Geometry: final body of the model. Coordinates: model frame, mm. Face numbers are marked on the shaded views. A direction names the side the tool comes from. Give positions to 0.01 mm unless a question says otherwise; leave off trailing zeros. Loops run counter-clockwise (first coordinate to the right, second up) from the corner with the lowest first, then second, coordinate; pieces in that order, holes last. Notation, with made-up numbers: (44, 48) - (67, 48) arc R25 ccw to (67, 81) - close; hole circle Ø4 at (75.25, 71). An arc over 180 degrees is marked (long way). Answer in a Markdown table with one row per item.
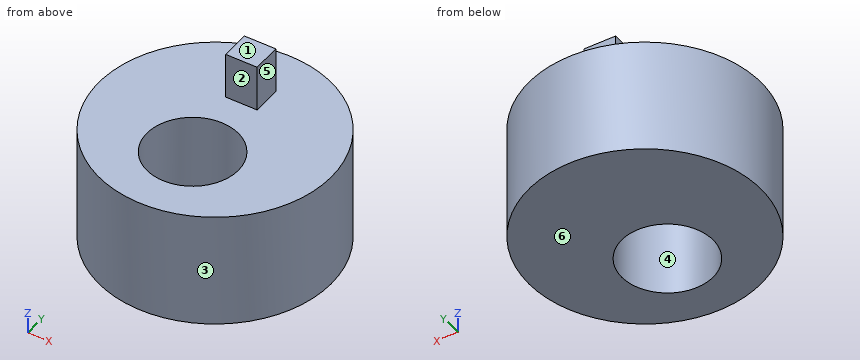
from build123d import *

# Parameters (mm, degrees)
SKETCH1_R           = 6.35
SKETCH1_R_2         = 2.499995
BOSS_EXTRUDE1_DEPTH = 6.35
SKETCH2_W           = 1.71989263
SKETCH2_H           = 1.584620177
BOSS_EXTRUDE2_DEPTH = 2.54


with BuildPart() as part:
    # Sketch1 → Boss-Extrude1 (new body)
    with BuildSketch(Plane.XY):
        Circle(SKETCH1_R)
        with Locations((0, -1.905)):
            Circle(SKETCH1_R_2, mode=Mode.SUBTRACT)
    extrude(amount=BOSS_EXTRUDE1_DEPTH)

    # Sketch2 → Boss-Extrude2 (add)
    with BuildSketch(Plane.XY.offset(6.35)):
        with Locations((-0.009662318, 3.043630217)):
            Rectangle(SKETCH2_W, SKETCH2_H)
    extrude(amount=BOSS_EXTRUDE2_DEPTH)


solid = part.part
Q1. Cut plane C-C (z = 6.75). Output: boundary loops of the cut face in (x, y), and give its area (3 significant figures).
Check values:
| item | result |
|---|---|
| outline | (-0.87, 2.25) - (0.85, 2.25) - (0.85, 3.84) - (-0.87, 3.84) - close |
| area | 2.73 mm² |
Q2. Cut plane D-D (y = 3.25). Output: boundary loops of the cut face in (x, z).
Check values:
| item | result |
|---|---|
| outline | (-5.46, 0) - (5.46, 0) - (5.46, 6.35) - (0.85, 6.35) - (0.85, 8.89) - (-0.87, 8.89) - (-0.87, 6.35) - (-5.46, 6.35) - close |
Q3. Draft query along X for the marked faces 3, 4, 5 and 6. Return one class per face: pulls with the +X half, pulls with the -X half, needs draft (parallel to the pull), parting line crosses it, or undercut.
Check values:
| item | result |
|---|---|
| face 3 | parting line crosses it |
| face 4 | undercut |
| face 5 | pulls with the +X half |
| face 6 | needs draft |
Q4. First-contact query: pin 1 (3 mm diameter, centred on x = -4.5, z = 5.5, fed in from -Y); pin 2 (0.9 mm diameter, centred on x = -0.5, z = 7.5, fed in from -Y); pin 3 (1.7 mm diameter, centred on y = 3, z = 7.5, fed in from -X). Flat tips, straight axial feed; report the tip coordinate or a pass-through.
Check values:
| item | result |
|---|---|
| pin 1 | y = -5.6 |
| pin 2 | y = 2.25 |
| pin 3 | x = -0.87 |
Q5. Cut plane A-A (x = 0). Output: boundary loops of the cut face in (y, z) (3 decimals), and give its area (3 significant figures).
Check values:
| item | result |
|---|---|
| outline | (-6.35, 0) - (-4.405, 0) - (-4.405, 6.35) - (-6.35, 6.35) - close; (0.595, 0) - (6.35, 0) - (6.35, 6.35) - (3.836, 6.35) - (3.836, 8.89) - (2.251, 8.89) - (2.251, 6.35) - (0.595, 6.35) - close |
| area | 52.9 mm² |
Q6. Cut plane B-B (y = -0.25). Output: boundary loops of the cut face in (x, z).
Check values:
| item | result |
|---|---|
| outline | (-6.35, 0) - (-1.87, 0) - (-1.87, 6.35) - (-6.35, 6.35) - close; (1.87, 0) - (6.35, 0) - (6.35, 6.35) - (1.87, 6.35) - close |
Q7. Reachability of the marked faces 1 and 2 from +Z, -Z, +X, -X, +Y, -Y: full face, straight path, thin tool, end or side. Return the list, or none.
Check values:
| item | result |
|---|---|
| face 1 | +Z, +X, -X, +Y, -Y |
| face 2 | +Z, +X, -X, -Y |
Q8. Material intervals for line 1 along Y through (x, z) = (0, 2) (3 decimals); line 2 along Z through (x, y) = (5.25, 0.75); line 3 along X through (y, z) = (-3, 2.25), sorted ascending.
Check values:
| item | result |
|---|---|
| line 1 | -6.35 to -4.405, 0.595 to 6.35 |
| line 2 | 0 to 6.35 |
| line 3 | -5.6 to -2.25, 2.25 to 5.6 |
